Check sheet for the drawn part. Datum: minimum x, y, z corner. Units: mm. A direction names the side the tool comes from. Round coordinates to 2 decimals unless told otherwise and drop trailing zeros. Write each loop counter-clockwise with the first axis right and the second up, starting at its lowest first coordinate (ties: lowest second). Pieces come first, ordered by that corner, then holes. Notation, with made-up numbers: (31.5, 53) - (60.5, 53) arc R10 ccw to (60.5, 58) - close; hole circle Ø11 at (33, -32.75). An arc over 180 degrees is marked (long way). Answer as a JSON object with one key per item and string values.
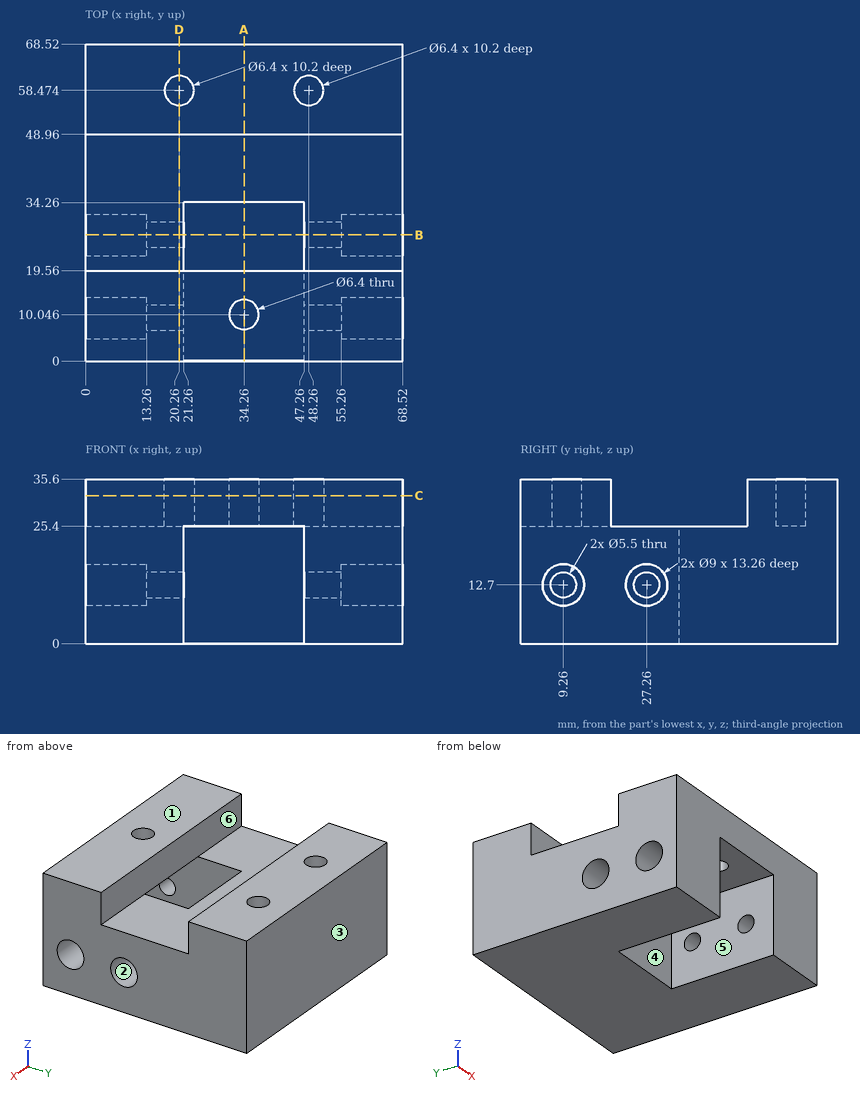
Q1. Section check A-A, the plane x = 34.26. Record the cut outline in (y, z).
Geometry check:
{"outline": "(0, 25.4) - (6.85, 25.4) - (6.85, 35.6) - (0, 35.6) - close; (13.25, 25.4) - (19.56, 25.4) - (19.56, 35.6) - (13.25, 35.6) - close; (34.26, 0) - (68.52, 0) - (68.52, 35.6) - (48.96, 35.6) - (48.96, 25.4) - (34.26, 25.4) - close"}
Q2. Section check C-C, the plane z = 32. Record the cut outline in (x, y), then the cut area to 3 significant figures.
Geometry check:
{"outline": "(0, 0) - (68.52, 0) - (68.52, 19.56) - (0, 19.56) - close; (0, 48.96) - (68.52, 48.96) - (68.52, 68.52) - (0, 68.52) - close; hole circle Ø6.4 at (20.26, 58.47); hole circle Ø6.4 at (34.26, 10.05); hole circle Ø6.4 at (48.26, 58.47)", "area": "2,580 mm2"}
Q3. Release check for a two-part mould opening along Z. For the marked faces 1, 2 and 3 record: released by +Z, released by -Z, zero draft, split by the parting line, or undercut.
Geometry check:
{"face 1": "released by +Z", "face 2": "undercut", "face 3": "zero draft"}
Q4. Section check B-B, the plane y = 27.26. Record the cut outline in (x, z).
Geometry check:
{"outline": "(0, 0) - (21.26, 0) - (21.26, 9.95) - (13.26, 9.95) - (13.26, 8.2) - (0, 8.2) - close; (0, 17.2) - (13.26, 17.2) - (13.26, 15.45) - (21.26, 15.45) - (21.26, 25.4) - (0, 25.4) - close; (47.26, 0) - (68.52, 0) - (68.52, 8.2) - (55.26, 8.2) - (55.26, 9.95) - (47.26, 9.95) - close; (47.26, 15.45) - (55.26, 15.45) - (55.26, 17.2) - (68.52, 17.2) - (68.52, 25.4) - (47.26, 25.4) - close"}
Q5. Set-up check for the marked faces 4, 5 and 6: record each of +Z, -Z, +X, -X, +Y, -Y from which the full face is reachable in a straight line by a thin tool's end or side.
Geometry check:
{"face 4": "+Z, -Z, -Y", "face 5": "-Z, -Y", "face 6": "+Z, +X, -X"}
Q6. Gauge pin test, flat ends, axial feed: P1, Ø6.5, axis at y = 9.26, z = 12.7, coming from the +X side; P2, Ø4.5, axis at y = 10, z = 11, coming from the -X side; P3, Ø14.5, axis at x = 32.5, y = 29, coming from the +Z side; P4, Ø5, axis at y = 9.26, z = 12.7, coming from the +X side. Record the tip position at first contact, or that the pin passes through.
Geometry check:
{"P1": "stops at x = 55.26", "P2": "stops at x = 13.26", "P3": "stops at z = 25.4", "P4": "passes through"}
Q7. Section check D-D, the plane x = 20.26. Record the cut outline in (y, z), then the cut area to 3 significant figures.
Geometry check:
{"outline": "(0, 0) - (68.52, 0) - (68.52, 35.6) - (61.67, 35.6) - (61.67, 25.4) - (55.27, 25.4) - (55.27, 35.6) - (48.96, 35.6) - (48.96, 25.4) - (19.56, 25.4) - (19.56, 35.6) - (0, 35.6) - close; hole circle Ø5.5 at (9.26, 12.7); hole circle Ø5.5 at (27.26, 12.7)", "area": "2,030 mm2"}
Q8. Material ranges on line 1 along Y through (x, z) = (20.26, 28); line 2 along Y through (x, z) = (3, 12.7); line 3 along Z through (x, y) = (60, 27), recorded low to high. Write a range as [from, to].
Geometry check:
{"line 1": "y = [0, 19.56], [48.96, 55.27], [61.67, 68.52]", "line 2": "y = [0, 4.76], [13.76, 22.76], [31.76, 68.52]", "line 3": "z = [0, 8.21], [17.19, 25.4]"}
